The drawing under review shows one solid part. Ordinate dimensions are in mm from its lowest x, y, z. A direction names the side the tool comes from. Coordinates: 2 decimals unless noted, no trailing zeros. Order: outer loops, then holes, each group sorted by start corner. A loop starts at its lowest first (then second) coordinate and runs counter-clockwise, first axis right, second up. Notation, with made-up numbers: (12, 10) -> (46, 10) arc R25 cw to (46, 44) -> close; hole circle Ø7 at (60, 29.5). An arc over 180 degrees is marked (long way). Use a Markdown table: item, result. Add a question column.
Q1. Add section B-B (y = 18). State the section outline as (x, z) points (1 decimal).
Q2. Add section D-D (y = 32). State the section outline as (x, z) points (1 decimal), then the cut area to 3 significant figures.
Q3. Wall thickness on probe 1 along Z at (x, y) = (109, 31); probe 2 along X at (y, z) = (20, 7.5) (1 decimal); probe 3 along Y at (x, z) = (109, 13.75): over which ranges is each line inside the solid? List them lowest first.
Q4. The part is to be moulded in two halves that separate along X. For the marked faces 1, 2 and 3, say which applies: pulls with the +X half, pulls with the -X half, needs draft (parallel to the pull), parting line crosses it, or undercut.
Q5. Add section A-A (x = 109). State the section outline as (y, z) points.
Q6. Insertion check: pin 1 (3 mm diameter, centred on x = 45.5, y = 19.5, fed in from -Z); pin 2 (1 mm diameter, centred on x = 108, y = 10, fed in from +Z); pin 3 (1.9 mm diameter, centred on x = 127.5, z = 6.5, fed in from +Y). Each pin has a flat end and moves straight along its axis. Give the tip position at first contact, or say it passes through.
Q7. Add section C-C (z = 11). State the section outline as (x, y) points (1 decimal).
Q8. Machinability: for the marked faces 4 and 5, which of the approach directions +Z, -Z, +X, -X, +Y, -Y give a long, thin tool a straight path to every point of the face, cutting with its end or side? Answer none if there is none.
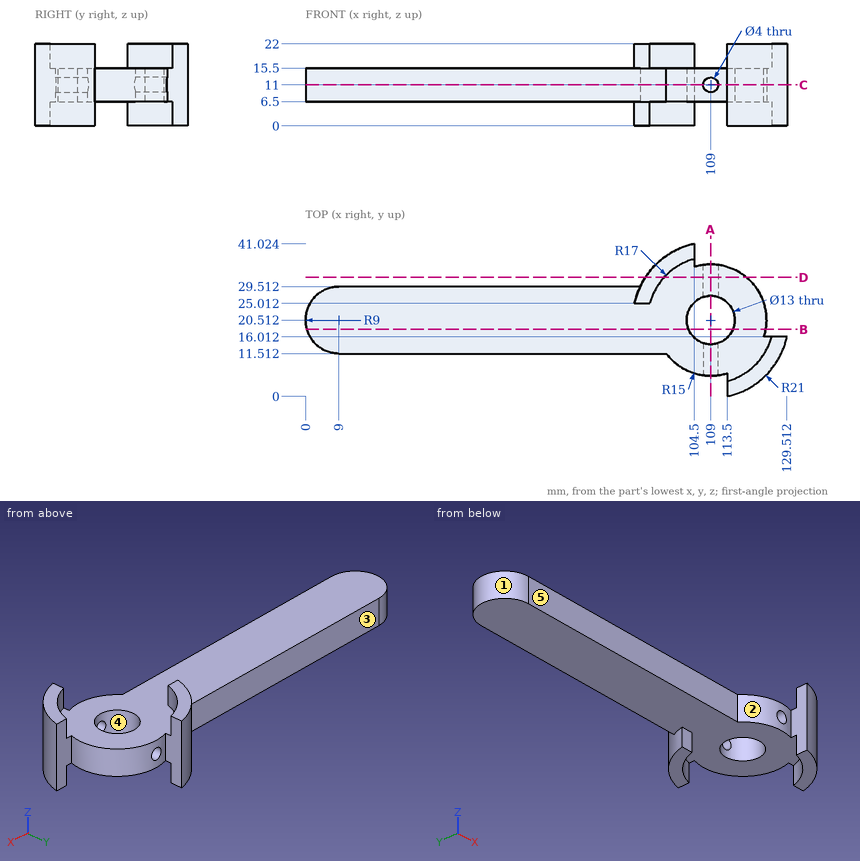
Established:
| question | item | result |
|---|---|---|
| 1 | outline | (0.4, 6.5) -> (103, 6.5) -> (103, 15.5) -> (0.4, 15.5) -> close; (115, 6.5) -> (123.8, 6.5) -> (123.8, 15.5) -> (115, 15.5) -> close |
| 2 | outline | (91.4, 0) -> (96.5, 0) -> (96.5, 6.5) -> (118.6, 6.5) -> (118.6, 15.5) -> (96.5, 15.5) -> (96.5, 22) -> (91.4, 22) -> close; hole circle Ø4 at (109, 11) |
| 2 | area | 298 mm^2 |
| 3 | probe 1 | 6.5 to 9, 13 to 15.5 |
| 3 | probe 2 | 0 to 102.5, 115.5 to 124 |
| 3 | probe 3 | 5.51 to 14.01, 27.01 to 35.51 |
| 4 | face 1 | pulls with the -X half |
| 4 | face 2 | undercut |
| 4 | face 3 | needs draft |
| 5 | outline | (5.51, 6.5) -> (14.01, 6.5) -> (14.01, 9) -> (5.51, 9) -> close; (5.51, 13) -> (14.01, 13) -> (14.01, 15.5) -> (5.51, 15.5) -> close; (27.01, 6.5) -> (35.51, 6.5) -> (35.51, 9) -> (27.01, 9) -> close; (27.01, 13) -> (35.51, 13) -> (35.51, 15.5) -> (27.01, 15.5) -> close |
| 6 | pin 1 | z = 6.5 |
| 6 | pin 2 | z = 15.5 |
| 6 | pin 3 | y = 16.01 |
| 7 | outline | (9, 11.5) -> (97, 11.5) arc R15 ccw to (107, 5.6) -> (107, 14.3) arc R6.5 cw to (107, 26.7) -> (107, 35.4) arc R15 ccw to (104.5, 34.8) -> (104.5, 41) arc R21 ccw to (90, 29.5) -> (9, 29.5) arc R9 ccw to start; (111, 5.6) arc R15 ccw to (113.5, 6.2) -> (113.5, 0) arc R21 ccw to (129.5, 16) -> (123.3, 16) arc R15 ccw to (111, 35.4) -> (111, 26.7) arc R6.5 cw to (111, 14.3) -> close |
| 8 | face 4 | +Z, -Z |
| 8 | face 5 | +Z, -Z, -X, -Y |
